Verification items for this drawing (mm, ordinates from the low corner). A direction names the side the tool comes from. Coordinates: 2 decimals unless noted, no trailing zeros. Write each loop counter-clockwise with the first axis right and the second up, starting at its lowest first coordinate (ties: lowest second). Pieces come first, ordered by that corner, then holes. Notation, with made-up numbers: (36, 25) -> (62, 25) arc R19 ccw to (62, 33) -> close; hole circle Ø6 at (19.25, 28.25). An arc over 180 degrees is marked (long way). One line per question, with ' | ' between items.
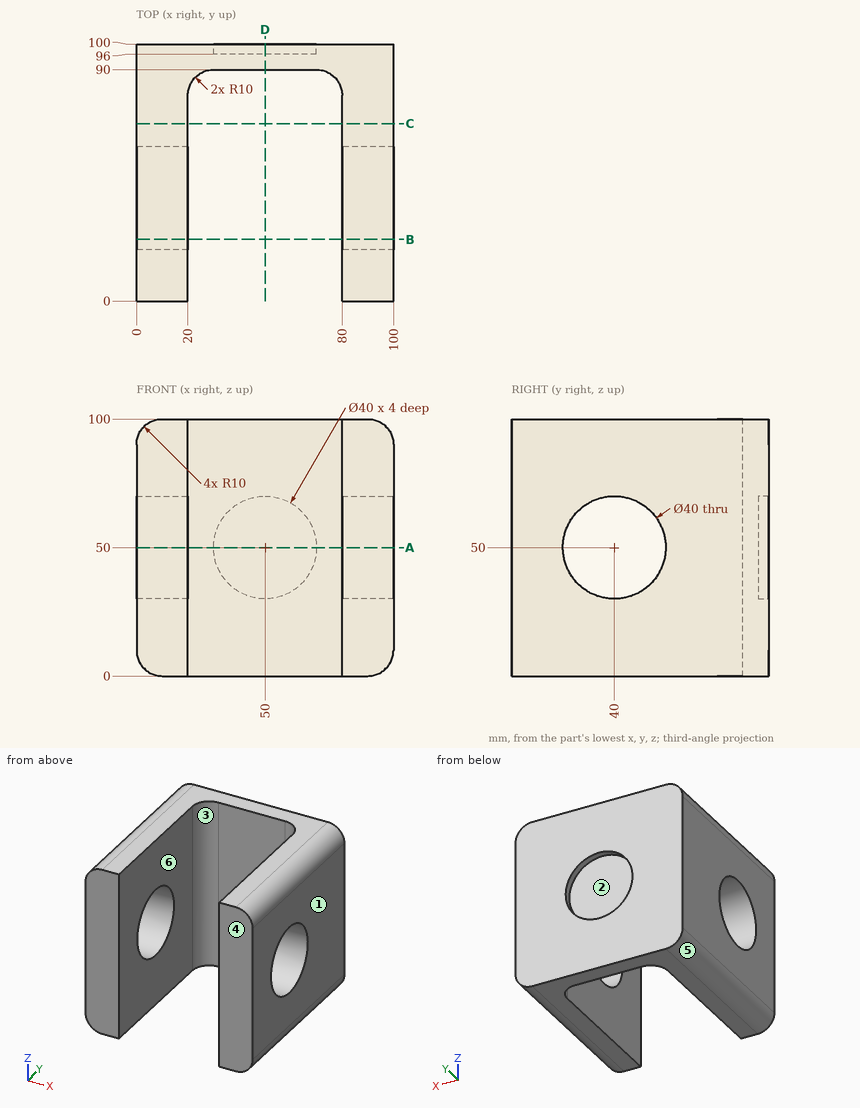
(1) Draft check along X on the marked faces 4, 5 and 6. Enter one of: pulls with the +X half, pulls with the -X half, needs draft (parallel to the pull), parting line crosses it, or undercut.
Answers below:
face 4: needs draft | face 5: pulls with the -X half | face 6: undercut
(2) Cross-section at D-D (x = 50). Record the cut outline in (y, z).
Answers below:
outline: (90, 0) -> (100, 0) -> (100, 30) -> (96, 30) -> (96, 70) -> (100, 70) -> (100, 100) -> (90, 100) -> close
(3) Cross-section at A-A (z = 50). Record the cut outline in (x, y), plus the area to 3 significant figures.
Answers below:
outline: (0, 0) -> (20, 0) -> (20, 20) -> (0, 20) -> close; (0, 60) -> (20, 60) -> (20, 80) arc R10 cw to (30, 90) -> (70, 90) arc R10 cw to (80, 80) -> (80, 60) -> (100, 60) -> (100, 100) -> (70, 100) -> (70, 96) -> (30, 96) -> (30, 100) -> (0, 100) -> close; (80, 0) -> (100, 0) -> (100, 20) -> (80, 20) -> close | area: 2,880 mm²
(4) Tool access check on the marked faces 1, 2 and 3. Record the directions out of +Z, -Z, +X, -X, +Y, -Y that give a thin tool (end or side, any length) a straight path to the whole face; none if there is none.
Answers below:
face 1: +Z, -Z, +X, +Y, -Y | face 2: +Y | face 3: +Z, -Z, -Y
(5) Cross-section at B-B (y = 24). Record the cut outline in (x, z).
Answers below:
outline: (0, 10) arc R10 ccw to (10, 0) -> (20, 0) -> (20, 38) -> (0, 38) -> close; (0, 62) -> (20, 62) -> (20, 100) -> (10, 100) arc R10 ccw to (0, 90) -> close; (80, 0) -> (90, 0) arc R10 ccw to (100, 10) -> (100, 38) -> (80, 38) -> close; (80, 62) -> (100, 62) -> (100, 90) arc R10 ccw to (90, 100) -> (80, 100) -> close
(6) Depth check by flat-ended pin: P1, Ø20, axis at x = 58, z = 65, coming from the -Y side; P2, Ø1.5, axis at x = 56, z = 50, coming from the +Y side; P3, Ø24, axis at y = 40, z = 50, coming from the +X side. Enter the tip coordinate at first touch or a pass-through.
Answers below:
P1: stops at y = 90 | P2: stops at y = 96 | P3: passes through
(7) Material ranges on line 1 (X direction, y = 98.3, z = 50); line 2 (X direction, y = 78, z = 87); line 3 (Y direction, x = 12.5, z = 50), recorded low to high.
Answers below:
line 1: x = 0 to 30, 70 to 100 | line 2: x = 0 to 20, 80 to 100 | line 3: y = 0 to 20, 60 to 100
(8) Cross-section at C-C (y = 69). Record the cut outline in (x, z).
Answers below:
outline: (0, 10) arc R10 ccw to (10, 0) -> (20, 0) -> (20, 100) -> (10, 100) arc R10 ccw to (0, 90) -> close; (80, 0) -> (90, 0) arc R10 ccw to (100, 10) -> (100, 90) arc R10 ccw to (90, 100) -> (80, 100) -> close
